Read the model definition and answer for the solid it produces. Units are mm, in the model's axes. Coordinates: 2 decimals unless noted, no trailing zeros. Loops run counter-clockwise (first coordinate to the right, second up) from the corner with the lowest first, then second, coordinate; pieces in that order, holes last. Notation, with made-up numbers: (52.25, -38.5) -> (99.25, -38.5) arc R12 ccw to (99.25, -34.5) -> close; hole circle Ø2 at (87, 78). An arc over 180 degrees is marked (long way). Answer as CSV lines item,"result".
```python
from build123d import *
from OCP.BRepFilletAPI import BRepFilletAPI_MakeChamfer

# Parameters (mm, degrees)
SKETCH1_W           = 4
SKETCH1_H           = 3
BOSS_EXTRUDE1_DEPTH = 0.77
SKETCH3_W           = 4
SKETCH3_H           = 3
BOSS_EXTRUDE2_DEPTH = 0.75
CHAMFER1_SIZE       = 0.75
CHAMFER2_SIZE       = 0.77
CHAMFER2_SIZE_2     = 0.04035399
SKETCH4_W           = 0.44
SKETCH4_H           = 0.38
BOSS_EXTRUDE3_DEPTH = 1.6
SKETCH5_W           = 0.54
SKETCH5_H           = 0.38
BOSS_EXTRUDE4_DEPTH = 0.7
SKETCH6_W           = 0.39
SKETCH6_H           = 0.38
BOSS_EXTRUDE5_DEPTH = 13
LPATTERN1_COUNT     = 3
LPATTERN1_PITCH     = 1.27


with BuildPart() as part:
    # Sketch1 → Boss-Extrude1 (new body)
    with BuildSketch(Plane(origin=(0, 0, 0), x_dir=(1, 0, 0), z_dir=(0, 1, 0))):
        with Locations((0, 1.5)):
            Rectangle(SKETCH1_W, SKETCH1_H)
    extrude(amount=BOSS_EXTRUDE1_DEPTH)

    # Sketch3 → Boss-Extrude2 (add)
    with BuildSketch(Plane.XZ):
        with Locations((0, -1.5)):
            Rectangle(SKETCH3_W, SKETCH3_H)
    extrude(amount=BOSS_EXTRUDE2_DEPTH)

    # Chamfer1
    chamfer1_edges = [part.edges().sort_by_distance(p)[0] for p in [
        (-2, -0.75, -1.5),
        (2, -0.75, -1.5),
    ]]
    chamfer(chamfer1_edges, length=CHAMFER1_SIZE)

    # Chamfer2
    chamfer2_edges_1 = [part.edges().sort_by_distance(p)[0] for p in [
        (-2, 0.77, -1.5),
    ]]
    chamfer2_side_1 = [part.faces().sort_by_distance(p)[0] for p in [
        (-2, 0.76919292, -1.5),
    ]]
    chamfer2_edges_2 = [part.edges().sort_by_distance(p)[0] for p in [
        (2, 0.77, -1.5),
    ]]
    chamfer2_side_2 = [part.faces().sort_by_distance(p)[0] for p in [
        (1.99919292, 0.77, -1.5),
    ]]
    chamfer2 = BRepFilletAPI_MakeChamfer(part.part.solid().wrapped)
    for e in chamfer2_edges_1:
        chamfer2.Add(CHAMFER2_SIZE - 0.0001, CHAMFER2_SIZE_2 - 0.0001, e.wrapped, chamfer2_side_1[0].wrapped)
    for e in chamfer2_edges_2:
        chamfer2.Add(CHAMFER2_SIZE_2 - 0.0001, CHAMFER2_SIZE - 0.0001, e.wrapped, chamfer2_side_2[0].wrapped)
    add(Compound.cast(chamfer2.Shape()), mode=Mode.REPLACE)  # a hair under: the kernel refuses the full size

    # Sketch4 → Boss-Extrude3 (add)
    with BuildSketch(Plane.XY):
        with Locations((-1.27, 0)):
            Rectangle(SKETCH4_W, SKETCH4_H)
    boss_extrude3 = extrude(amount=BOSS_EXTRUDE3_DEPTH)

    # Sketch5 → Boss-Extrude4 (add)
    with BuildSketch(Plane.XY.offset(1.6)):
        with Locations((-1.27, 0)):
            Rectangle(SKETCH5_W, SKETCH5_H)
    boss_extrude4 = extrude(amount=BOSS_EXTRUDE4_DEPTH)

    # Sketch6 → Boss-Extrude5 (add)
    with BuildSketch(Plane.XY.offset(2.3)):
        with Locations((-1.27, 0)):
            Rectangle(SKETCH6_W, SKETCH6_H)
    boss_extrude5 = extrude(amount=BOSS_EXTRUDE5_DEPTH)

    # LPattern1: Boss-Extrude3, Boss-Extrude4, Boss-Extrude5 ×3
    with Locations(*[(i * LPATTERN1_PITCH, 0, 0) for i in range(1, LPATTERN1_COUNT)]):
        add(boss_extrude3)
        add(boss_extrude4)
        add(boss_extrude5)


solid = part.part
```
Q1. For a pull along X with two mould halves and no side action, classify faces 1 (the face through (0, 0.4, 0)), 2 (the face through (0, -0.75, -1)) as pulls with the +X half, pulls with the -X half, needs draft (parallel to the pull), parting line crosses it, or undercut.
Results:
face 1,"undercut"
face 2,"needs draft"
Q2. A cutting plane is placed at B-B, the plane y = -0.35. Write down the section's boundary in (x, z).
Results:
outline,"(-1.65, -3) -> (1.65, -3) -> (1.65, 0) -> (-1.65, 0) -> close"
Q3. A cutting plane is placed at C-C, the plane x = -0.45. Write down the section's boundary in (y, z).
Results:
outline,"(-0.75, -3) -> (0.77, -3) -> (0.77, 0) -> (-0.75, 0) -> close"
Q4. A cutting plane is placed at A-A, the plane z = 4.25. Write down the section's boundary in (x, y) (3 decimals), and give its area (3 significant figures).
Results:
outline,"(-1.465, -0.19) -> (-1.075, -0.19) -> (-1.075, 0.19) -> (-1.465, 0.19) -> close; (-0.195, -0.19) -> (0.195, -0.19) -> (0.195, 0.19) -> (-0.195, 0.19) -> close; (1.075, -0.19) -> (1.465, -0.19) -> (1.465, 0.19) -> (1.075, 0.19) -> close"
area,"0.445 mm²"
Q5. Find the intervals of material crossed by probe 1 along X at (y, z) = (0.05, 0.75); probe 2 along X at (y, z) = (-0.15, 12) (3 decimals); probe 3 along Z at (x, y) = (1.45, 0.7), in increasing order. Write a range as [from, to].
Results:
probe 1,"x = [-1.49, -1.05], [-0.22, 0.22], [1.05, 1.49]"
probe 2,"x = [-1.465, -1.075], [-0.195, 0.195], [1.075, 1.465]"
probe 3,"z = [-3, 0]"
